Geometry: final body of the model. Coordinates: model frame, mm. Coordinates: 2 decimals unless noted, no trailing zeros. Order: outer loops, then holes, each group sorted by start corner. A loop starts at its lowest first (then second) coordinate and runs counter-clockwise, first axis right, second up. Notation, with made-up numbers: M -12.5,9.5 L 2.5,9.5 A11 cw 2.5,27.5 Z; hole C -31.75,33.5 d11. An arc over 180 degrees is marked long. Write item = value, one per line.
from build123d import *

# Parameters (mm, degrees)
F1_DEPTH = 6.35
F3_DEPTH = 15.24
F4_W     = 515.874
F4_H     = 352.143454
F5_DEPTH = 9.9822
F6_W     = 503.174003
F6_H     = 339.443454
F7_DEPTH = 16.3332


with BuildPart() as f1:
    # F0 (on Front) → F1 (new body)
    with BuildSketch(Plane.XZ):
        Polygon((0, 95.25), (0, 0), (535.559, 0), (535.559, 95.25), (548.259, 95.25), (548.259, 133.35), (535.559, 133.35), (535.559, 228.635954), (548.259, 228.635954), (548.259, 266.735954), (535.559, 266.735954), (535.559, 361.985954), (433.959, 361.985954), (433.959, 374.685954), (383.159, 374.685954), (383.159, 361.985954), (152.4, 361.985954), (152.4, 374.685954), (101.6, 374.685954), (101.6, 361.985954), (0, 361.985954), (0, 266.735954), (-12.7, 266.735954), (-12.7, 228.635954), (0, 228.635954), (0, 133.35), (-12.7, 133.35), (-12.7, 95.25), align=None)
    extrude(amount=F1_DEPTH)

    # F2 (on face) → F3 (join)
    with BuildSketch(Plane(origin=(0, 0, 0), x_dir=(-1, 0, 0), z_dir=(0, 1, 0))):
        Polygon((0, 361.985954), (-535.559, 361.985954), (-535.559, 359.445954), (-535.559, 354.683454), (-535.559, 352.143454), (-535.559, 0), (-533.019, 0), (-533.019, 352.143454), (-533.019, 354.683454), (-533.019, 359.445954), (-2.54, 359.445954), (0, 359.445954), align=None)
        Polygon((0, 352.143454), (0, 354.683454), (-2.54, 354.683454), (-2.54, 352.143454), (-2.54, 0), (0, 0), align=None)
        Polygon((-528.2565, 352.143454), (-528.2565, 0), (-525.7165, 0), (-525.7165, 352.143454), (-9.8425, 352.143454), (-9.8425, 0), (-7.3025, 0), (-7.3025, 352.143454), (-7.3025, 354.683454), (-528.2565, 354.683454), align=None)
    extrude(amount=F3_DEPTH)

    # F4 (on face) → F5 (join)
    with BuildSketch(Plane(origin=(0, 0, 0), x_dir=(-1, 0, 0), z_dir=(0, 1, 0))):
        with Locations((-267.7795, 176.071727)):
            Rectangle(F4_W, F4_H)
    extrude(amount=F5_DEPTH)

    # F6 (on face) → F7 (cut, through all)
    with BuildSketch(Plane(origin=(0, 9.9822, 0), x_dir=(-1, 0, 0), z_dir=(0, 1, 0))):
        with Locations((-267.779501, 176.071727)):
            Rectangle(F6_W, F6_H)
    extrude(amount=-F7_DEPTH, mode=Mode.SUBTRACT)


solid = f1.part
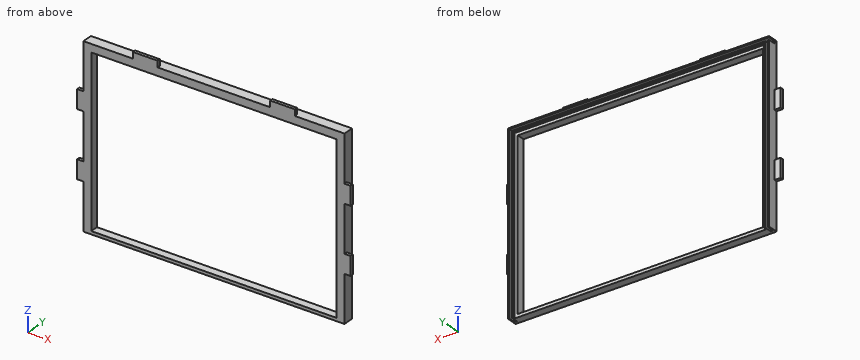
1) Pin query (flat end, axial travel): pin 1 (12 mm diameter, centred on y = 8.5, z = 250.5, fed in from -X); pin 2 (6.5 mm diameter, centred on x = 403, z = 367, fed in from +Y); pin 3 (4 mm diameter, centred on y = 0.5, z = 199, fed in from +X). Return the tip coordinate at first contact, or that it passes through.
Numbers:
pin_1 = 0
pin_2 = 0
pin_3 = 535.56
2) Section C-C, the plane y = 4.5. Return loops of the section in (x, z).
Numbers:
outline = M 0,0 L 2.54,0 L 2.54,354.68 L 0,354.68 Z; M 0,359.45 L 533.02,359.45 L 533.02,0 L 535.56,0 L 535.56,361.99 L 0,361.99 Z; M 7.3,0 L 528.26,0 L 528.26,354.68 L 7.3,354.68 Z; hole M 16.19,6.35 L 519.37,6.35 L 519.37,345.79 L 16.19,345.79 Z
3) Section A-A, the plane z = 177. Return loops of the section in (x, y), and give its area (3 significant figures).
Numbers:
outline = M 0,-6.35 L 16.19,-6.35 L 16.19,9.98 L 9.84,9.98 L 9.84,15.24 L 7.3,15.24 L 7.3,0 L 2.54,0 L 2.54,15.24 L 0,15.24 Z; M 519.37,-6.35 L 535.56,-6.35 L 535.56,15.24 L 533.02,15.24 L 533.02,0 L 528.26,0 L 528.26,15.24 L 525.72,15.24 L 525.72,9.98 L 519.37,9.98 Z
area = 487 mm²
4) Line query: L1, parallel to Z at x = 153, y = 5.75; L2, parallel to X at y = 11.75, z = 40; L3, parallel to Z at x = 424, y = -0.5. Output: solid intervals per line, ascending.
Numbers:
L1 = 0 to 6.35, 345.79 to 354.68, 359.45 to 361.99
L2 = 0 to 2.54, 7.3 to 9.84, 525.72 to 528.26, 533.02 to 535.56
L3 = 0 to 6.35, 345.79 to 374.69
5) Section D-D, the plane z = 104.5. Return loops of the section in (x, y).
Numbers:
outline = M -12.7,-6.35 L 16.19,-6.35 L 16.19,9.98 L 9.84,9.98 L 9.84,15.24 L 7.3,15.24 L 7.3,0 L 2.54,0 L 2.54,15.24 L 0,15.24 L 0,0 L -12.7,0 Z; M 519.37,-6.35 L 548.26,-6.35 L 548.26,0 L 535.56,0 L 535.56,15.24 L 533.02,15.24 L 533.02,0 L 528.26,0 L 528.26,15.24 L 525.72,15.24 L 525.72,9.98 L 519.37,9.98 Z
6) Section B-B, the plane x = 464. Return loops of the section in (y, z).
Numbers:
outline = M -6.35,0 L 9.98,0 L 9.98,6.35 L -6.35,6.35 Z; M -6.35,345.79 L 9.98,345.79 L 9.98,352.14 L 15.24,352.14 L 15.24,354.68 L 0,354.68 L 0,359.45 L 15.24,359.45 L 15.24,361.99 L -6.35,361.99 Z
